Drawing for the job (mm, zero at the part's lowest x, y, z). A direction names the side the tool comes from. Coordinates: 2 decimals unless noted, no trailing zeros. Order: outer loops, then holes, each group sorted by start corner. A loop starts at its lowest first (then second) coordinate and runs counter-clockwise, first axis right, second up. Notation, with made-up numbers: (-19.75, 44) -> (-9.75, 44) arc R30 cw to (-9.75, 79) -> close; hole circle Ø3 at (34, 36). An arc over 180 degrees is marked (long way). Write each question's results on one line, items separated by ' | '.
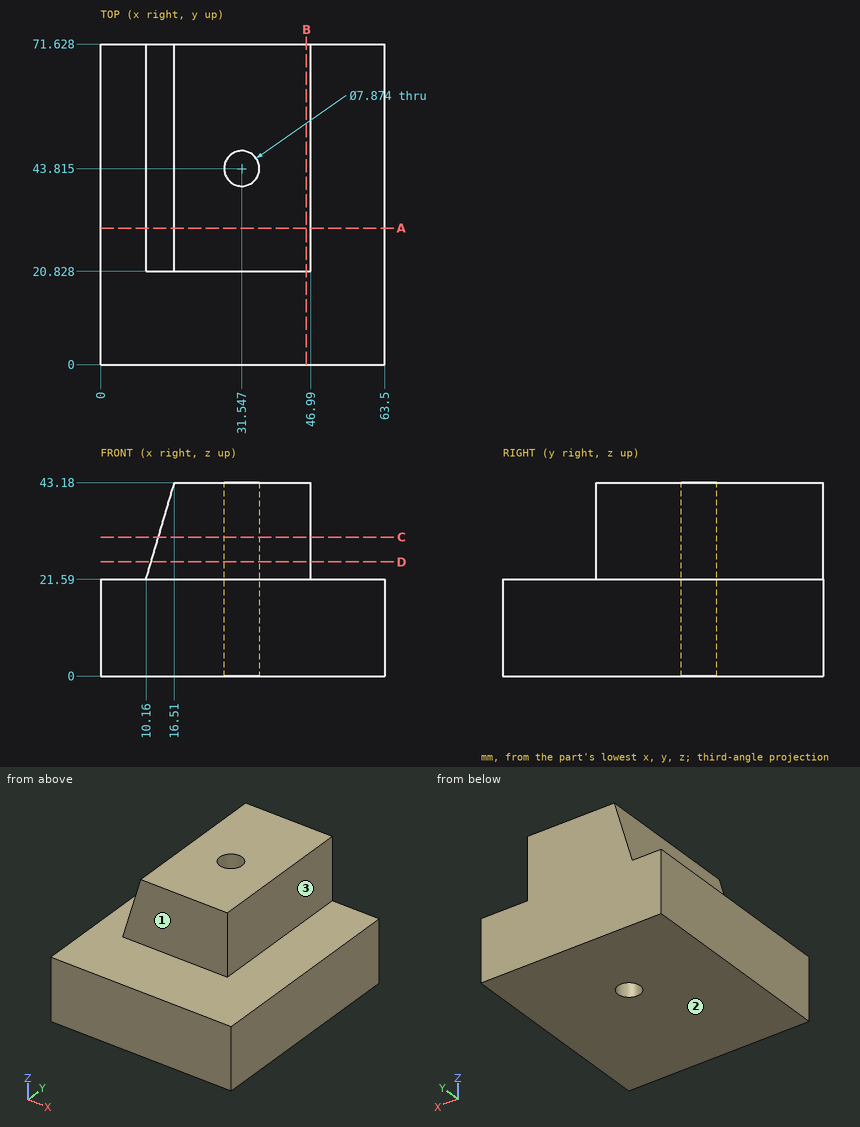
Item 1: Drill centre lines: line 1 (Y direction, x = 45, z = 37); line 2 (Z direction, x = 30.5, y = 15.5); line 3 (X direction, y = 43.5, z = 24.5). Where is each one in solid material? Low to high. Write a range as from..to.
Answer:
line 1: y = 20.83..71.63 | line 2: z = 0..21.59 | line 3: x = 11.02..27.62, 35.47..46.99
Item 2: Slice it at C-C, the plane z = 31. List the corners of the cut face in (x, y) (1 decimal).
Answer:
outline: (12.9, 20.8) -> (47, 20.8) -> (47, 71.6) -> (12.9, 71.6) -> close; hole circle Ø7.9 at (31.5, 43.8)
Item 3: Slice it at D-D, the plane z = 25.5. List the corners of the cut face in (x, y) (3 decimals).
Answer:
outline: (11.31, 20.828) -> (46.99, 20.828) -> (46.99, 71.628) -> (11.31, 71.628) -> close; hole circle Ø7.874 at (31.547, 43.815)
Item 4: Pin check, flat tips, straight feed: pin 1 (6.5 mm diameter, centred on y = 48, z = 37, fed in from +X); pin 2 (5 mm diameter, centred on x = 19, z = 29, fed in from -Y); pin 3 (10 mm diameter, centred on y = 13.5, z = 27.5, fed in from +X). Stop position of each tip, or through.
Answer:
pin 1: stops at x = 46.99 | pin 2: stops at y = 20.83 | pin 3: passes through
Item 5: Slice it at B-B, the plane x = 46. List the corners of the cut face in (y, z).
Answer:
outline: (0, 0) -> (71.63, 0) -> (71.63, 43.18) -> (20.83, 43.18) -> (20.83, 21.59) -> (0, 21.59) -> close
Item 6: Slice it at A-A, the plane y = 30.5. List the corners of the cut face in (x, z).
Answer:
outline: (0, 0) -> (63.5, 0) -> (63.5, 21.59) -> (46.99, 21.59) -> (46.99, 43.18) -> (16.51, 43.18) -> (10.16, 21.59) -> (0, 21.59) -> close
Item 7: Tool access for the marked faces 1, 2 and 3: list every direction of +Z, -Z, +X, -X, +Y, -Y with a clear straight run to the whole face (end or side of a thin tool).
Answer:
face 1: +Z, +X, -X, -Y | face 2: -Z, +X, -X, +Y, -Y | face 3: +Z, +X, +Y, -Y
